The model under review builds one solid part; all positions refer to its coordinate system, in mm. A direction names the side the tool comes from. Give positions to 0.01 mm unless a question says otherwise; leave off trailing zeros. Write each loop counter-clockwise with the first axis right and the second up, starting at its lowest first coordinate (ties: lowest second). Pieces come first, ordered by that corner, then holes. Notation, with made-up numbers: (56, -29.75) - (83, -29.75) arc R11 ccw to (83, -20.75) - close; hole circle Ø3 at (-28, 76.5). An arc over 180 degrees is marked (long way). Write item = value, one per line.
```python
from build123d import *

# Parameters (mm, degrees)
SKETCH_1_W          = 63.552014958
SKETCH_1_H          = 75.18168128
EXTRUDE_1_DEPTH     = 2
CUT_EXTRUDE_3_DEPTH = 2
CUT_EXTRUDE_4_DEPTH = 2
SKETCH_2_R          = 2.6
SKETCH_2_R_2        = 1.5
EXTRUDE_2_DEPTH     = 6


with BuildPart() as part:
    # 草图1 → 凸台-拉伸1 (new body)
    with BuildSketch(Plane(origin=(0, 0, 0), x_dir=(0, 0, -1), z_dir=(1, 0, 0))):
        with Locations((-6.130256719, 2.766182452)):
            Rectangle(SKETCH_1_W, SKETCH_1_H)
    extrude(amount=EXTRUDE_1_DEPTH)

    # 草图3 → 切除-拉伸3 (cut)
    with BuildSketch(Plane(origin=(2, 0, 0), x_dir=(0, 0, -1), z_dir=(1, 0, 0))):
        Polygon((-37.906264198, -19.734560887), (-37.906264198, 40.357023092), (25.64575076, 40.357023092), (25.64575076, -13.40384327), (25.64575076, -23.166877668), (25.64575076, -34.824658188), (-37.906264198, -34.824658188), (-37.906264198, -23.166877668), align=None)
        Polygon((3.861598797, 38.157182144), (-33.05487502, -19.734560887), (-33.05487502, -23.166877668), (24.455499481, -23.166877668), (24.455499481, -13.40384327), (10.344863827, 38.157182144), align=None, mode=Mode.SUBTRACT)
    extrude(amount=-CUT_EXTRUDE_3_DEPTH, mode=Mode.SUBTRACT)

    # 草图4 → 切除-拉伸4 (cut)
    with BuildSketch(Plane(origin=(2, 0, 0), x_dir=(0, 0, -1), z_dir=(1, 0, 0))):
        Polygon((0.937037541, 25.644128731), (-20.204452885, -12.953479978), (16.800310672, -12.953479978), (6.235289924, 25.644128731), align=None)
    extrude(amount=-CUT_EXTRUDE_4_DEPTH, mode=Mode.SUBTRACT)

    # 草图2 → 凸台-拉伸2 (add)
    with BuildSketch(Plane(origin=(2, 0, 0), x_dir=(0, 0, -1), z_dir=(1, 0, 0))):
        with Locations((6.295781653, 33.876700988)):
            Circle(SKETCH_2_R)
        with Locations((6.295781653, 33.876700988)):
            Circle(SKETCH_2_R_2, mode=Mode.SUBTRACT)
        with Locations((-27.006264198, -18.064263021)):
            Circle(SKETCH_2_R)
        with Locations((-27.006264198, -18.064263021)):
            Circle(SKETCH_2_R_2, mode=Mode.SUBTRACT)
        with Locations((21.283382726, -17.064263021)):
            Circle(SKETCH_2_R)
        with Locations((21.283382726, -17.064263021)):
            Circle(SKETCH_2_R_2, mode=Mode.SUBTRACT)
    extrude(amount=-EXTRUDE_2_DEPTH)


solid = part.part
```
1. Take a section at C-C on z = 8.5. Give the boundary of the cut face in (x, y).
Findings below:
outline = (0, -23.17) - (2, -23.17) - (2, -12.95) - (0, -12.95) - close; (0, 8.42) - (2, 8.42) - (2, 18.77) - (0, 18.77) - close
2. Machinability: for faces 5 (the flat face through (0, 34, -6)), 6 (the flat face through (1, -21, 33.055)), 7 (the flat face through (1.014, 6.616, 9.486)), which of the approach directions +Z, -Z, +X, -X, +Y, -Y give a long, thin tool a straight path to every point of the face, cutting with its end or side? Answer none if there is none.
Findings below:
face_5 = -X
face_6 = +Z, +X, -X, +Y, -Y
face_7 = +X, -X
3. Draft analysis for pull direction Y (two halves, no side actions). For faces 1 (the flat face through (1, -12.953, 2)), 2 (the cylindrical face through (-1.972, -16.95, -18.686)), 3 (the flat face through (1, 38.157, -7)), 4 (the flat face through (1, 25.644, -4)), state which applies: +Y half, -Y half, draft (parallel to the pull), parting line (faces both ways), or undercut.
Findings below:
face_1 = undercut
face_2 = parting line
face_3 = +Y half
face_4 = undercut
4. For line 1 (Y direction, x = 0.2, z = -4.5); line 2 (Y direction, x = -2.05, z = -21.5); line 3 (Z direction, x = 1, y = 3), list the stretches that pass through material, from the lowest coordinate up. Write a range as from..to.
Findings below:
line_1 = -23.17..-12.95, 25.64..38.16
line_2 = -19.66..-18.55, -15.58..-14.47
line_3 = -19.97..-12.43, 11.47..18.56
5. Take a section at D-D on x = -3.3. Give the boundary of the cut face in (y, z).
Findings below:
outline = circle Ø5.2 at (-18.06, 27.01); circle Ø5.2 at (-17.06, -21.28); circle Ø5.2 at (33.88, -6.3); hole circle Ø3 at (-18.06, 27.01); hole circle Ø3 at (-17.06, -21.28); hole circle Ø3 at (33.88, -6.3)
6. Take a section at B-B on y = -6. Give the boundary of the cut face in (x, z).
Findings below:
outline = (0, -22.43) - (2, -22.43) - (2, -14.9) - (0, -14.9) - close; (0, 16.4) - (2, 16.4) - (2, 24.3) - (0, 24.3) - close
7. Insertion check: P1, Ø1.5, axis at y = -18, z = 27, coming from the -X side. The pin has a flat end and moves straight along its axis. Give the tip position at first contact, or say it passes through.
Findings below:
P1 = 0
8. Take a section at A-A on x = 1. Give the boundary of the cut face in (y, z), and give its area (3 significant figures).
Findings below:
outline = (-23.17, -24.46) - (-13.4, -24.46) - (38.16, -10.34) - (38.16, -3.86) - (-19.73, 33.05) - (-23.17, 33.05) - close; hole (-12.95, -16.8) - (25.64, -6.24) - (25.64, -0.94) - (-12.95, 20.2) - close
area = 1,280 mm²
